Read the model definition and answer for the solid it produces. Units are mm, in the model's axes. A direction names the side the tool comes from. Give positions to 0.01 mm unless a question says otherwise; leave off trailing zeros. Order: outer loops, then holes, each group sorted by start corner. A loop starts at its lowest first (then second) coordinate and runs counter-clockwise, first axis right, second up. Notation, with made-up numbers: (25, -20.5) -> (68, -20.5) arc R15 cw to (68, -7.5) -> close; hole circle Ø4 at (46.5, 15). An arc over 180 degrees is marked (long way). Use one line per item in the form item = value.
Autodesk Inventor part; units mm, degrees
ref_plane "YZ Plane" through (0, 0, 0) normal (1, 0, 0) x (0, 1, 0)
ref_plane "XZ Plane" through (0, 0, 0) normal (0, 1, 0) x (-1, 0, 0)
ref_plane "XY Plane" through (0, 0, 0) normal (0, 0, 1) x (1, 0, 0)
sketch "Sketch1" plane through (0, 0, 0) normal (0, 0, 1) x (1, 0, 0)
  line L0 (0, 0) -> (0, 2.5)
  line L1 (-2.5, 0) -> (-2.5, 2)
  line L2 (-2.5, 2) -> (-3, 2.5)
  line L3 (-3, 2.5) -> (-4.3, 2.5)
  line L4 (-4.3, 2.5) -> (-4.3, 2.3)
  line L5 (-4.3, 2.3) -> (-6.85, 2.3)
  line L6 (-6.85, 2.3) -> (-6.85, 2.5)
  line L7 (-6.85, 2.5) -> (-7.6465, 2.5)
  line L8 (-7.6465, 2.5) -> (-8, 2.1465)
  line L9 (-8, 2.1465) -> (-8, 0)
  line L10 (-8, 0) -> (-2.5, 0)
  dimension "d9" = 2.5
  dimension "d19" = 2.5
  dimension "d20" = 0.2
  dimension "d21" = 5
  dimension "d22" = 6
  dimension "d23" = 8.6
  dimension "d24" = 13.7
  dimension "d26" = 16
  dimension "d27" = 135
  dimension "d29" = 0.5
  dimension "d30" = 15.293
revolve "Revolution1" add sketch "Sketch1" angle 360 about axis through (0, 0, 0) along (0, 1, 0)
mirror "Mirror1" about plane through (-5.25, 0, 0) normal (0, -1, 0) of "Revolution1"
equation "\"d19\" = d9"
properties part number "625 2RS Bearing"
Item 1: Straight lines are drawn through the part: L1, parallel to Z at x = 0, y = 0.35; L2, parallel to Y at x = 1.25, z = -5.75; L3, parallel to Z at x = 0, y = -2.4. For each, find the intervals that lie inside material, in ascending order. Write a range as from..to.
Checks:
L1 = -8..-2.5, 2.5..8
L2 = -2.3..2.3
L3 = -7.75..-6.85, -4.3..-2.9, 2.9..4.3, 6.85..7.75
Item 2: Given pin 1 Ø3 at (x, y) = (-3, 1) entering from -Z; pin 2 Ø1.5 at (y, z) = (-0.5, -6) entering from +X; pin 3 Ø3 at (x, z) = (0, 0) entering from -Y, each flat-ended and moving along its own axis, determine where each tip first touches the part or whether it passes through.
Checks:
pin_1 = -7.86
pin_2 = 6.04
pin_3 = through
Item 3: Which of the six approach directions +Z, -Z, +X, -X, +Y, -Y give full straight-line access (tool end or side, diameter ignored) to faces 4 (the flat face through (0.1, 2.3, -4.5)), 5 (the flat face through (-0.1, -2.3, -4.5)), 6 (the flat face through (-3, -2.5, -1))?
Checks:
face_4 = +Y
face_5 = -Y
face_6 = +Z, -Z, +X, -X, -Y
Item 4: The part is cut by section B-B on y = 1.1. Give the vertices of the cut face in (x, z), and give its area (3 significant figures).
Checks:
outline = circle Ø16 at (0, 0); hole circle Ø5 at (0, 0)
area = 181 mm²
Item 5: Determine the mould class of faces 1 (the flat face through (7, 2.5, -1)), 2 (the cylindrical face through (1.73, -0.03, 7.81)), 3 (the cylindrical face through (0.54, -0.03, 2.44)) for opening direction Z: +Z half, -Z half, draft (parallel to the pull), parting line (faces both ways), or undercut.
Checks:
face_1 = draft
face_2 = parting line
face_3 = undercut
